The listing builds one solid part. Answer for the finished solid, in the listing's coordinates (mm). Give positions to 0.01 mm unless a question says otherwise; leave off trailing zeros. Write each loop counter-clockwise with the first axis right and the second up, starting at its lowest first coordinate (ties: lowest second). Pieces come first, ordered by that corner, then holes. Notation, with made-up numbers: (46, 44.5) - (103, 44.5) arc R28 cw to (103, 77.5) - close; hole circle Ø10 at (47, 89). An arc over 180 degrees is marked (long way). Answer as CSV lines item,"result". Start each with the question number.
(1) Each of these flat-tipped pins is pushed along its axis until it touches: pin 1 Ø0.7 at (x, z) = (15.5, 2) entering from -Y; pin 2 Ø0.7 at (x, z) = (16, 2) entering from +Y; pin 3 Ø1.5 at (y, z) = (-2.5, 1.5) entering from +X; pin 4 Ø1 at (y, z) = (5.5, 1) entering from -X. Where does it stop, or does it pass through?
(2) Find section B-B (y = -4.75). Write down the section's boundary in (x, z), then the cut area to 3 significant figures.
(3) Straight lines are drawn through the part: probe 1 along X at (y, z) = (1, 1.95); probe 2 along X at (y, z) = (-1, 0.65); probe 3 along Z at (x, y) = (56, -5.5). For each, find the intervals that lie inside material, in ascending order.
(4) Find section A-A (x = 30.5). Write down the section's boundary in (y, z), then the cut area to 3 significant figures.
(5) Find section C-C (x = 48). Write down the section's boundary in (y, z), then the cut area to 3 significant figures.
from build123d import *

# Parameters (mm, degrees)
SKETCH_1_W                      = 90
SKETCH_1_H                      = 15
EXTRUDE_1_DEPTH                 = 2
SKETCH_2_W                      = 3
SKETCH_2_H                      = 3
EXTRUDE_2_DEPTH                 = 1
EXTRUDE_3_DEPTH                 = 2
CUT_EXTRUDE_1_REACH             = 84.878
CUT_EXTRUDE_1_DIRECTION_2_REACH = 84.878
FILLET_1_R                      = 0.1
FILLET_1_OF_MIRROR_1_R          = 0.1
FILLET_1_OF_MIRROR_3_R          = 0.1
FILLET_2_R                      = 0.2


# Read off the part's stored shape, not the designer's step: the mirror step
with BuildPart() as part:
    # Sketch 1 → Extrude 1 (new body)
    with BuildSketch(Plane.XY):
        with Locations((37.5, 0)):
            Rectangle(SKETCH_1_W, SKETCH_1_H)
    extrude(amount=-EXTRUDE_1_DEPTH)

    # Sketch 2 → Extrude 2 (add)
    with BuildSketch(Plane.XY):
        Rectangle(SKETCH_2_W, SKETCH_2_H)
    extrude_2 = extrude(amount=EXTRUDE_2_DEPTH)

    # Sketch 3 → Extrude 3 (add, symmetric)
    with BuildSketch(Plane(origin=(0, 0, 0), x_dir=(1, 0, 0), z_dir=(0, 1, 0))):
        with BuildLine():
            Line((-1.95, -2.5), (1.95, -2.5))
            Line((1.95, -2.5), (1.95, -1.555590279))
            ThreePointArc((1.95, -1.555590279), (1.780042303, -1.088161527), (1.5, -0.677124344))
            Line((1.5, -0.677124344), (-1.5, -0.677124344))
            ThreePointArc((-1.5, -0.677124344), (-1.780042303, -1.088161527), (-1.95, -1.555590279))
            Line((-1.95, -1.555590279), (-1.95, -2.5))
        make_face()
    extrude_3 = extrude(amount=EXTRUDE_3_DEPTH, both=True)

    # Sketch 4 → Cut-Extrude 1 (cut, up to next)
    with BuildSketch(Plane(origin=(0, 0, 0), x_dir=(0, 0, -1), z_dir=(1, 0, 0)), mode=Mode.PRIVATE) as cut_extrude_1_sk1:
        with BuildLine():
            Line((-2.5, 1.95), (-1.555590279, 1.95))
            ThreePointArc((-1.555590279, 1.95), (-1.088161527, 1.780042303), (-0.677124344, 1.5))
            Line((-0.677124344, 1.5), (-0.677124344, 2))
            Line((-0.677124344, 2), (-2.5, 2))
            Line((-2.5, 2), (-2.5, 1.95))
        make_face()
    cut_extrude_1_tool1 = extrude(cut_extrude_1_sk1.sketch, amount=-CUT_EXTRUDE_1_REACH, mode=Mode.PRIVATE) & part.part
    # Sketch 4 → Cut-Extrude 1 (cut, up to next)
    with BuildSketch(Plane(origin=(0, 0, 0), x_dir=(0, 0, -1), z_dir=(1, 0, 0)), mode=Mode.PRIVATE) as cut_extrude_1_sk2:
        with BuildLine():
            Line((-2.5, -2), (-0.677124344, -2))
            Line((-0.677124344, -2), (-0.677124344, -1.5))
            ThreePointArc((-0.677124344, -1.5), (-1.088161527, -1.780042303), (-1.555590279, -1.95))
            Line((-1.555590279, -1.95), (-2.5, -1.95))
            Line((-2.5, -1.95), (-2.5, -2))
        make_face()
    cut_extrude_1_tool2 = extrude(cut_extrude_1_sk2.sketch, amount=-CUT_EXTRUDE_1_REACH, mode=Mode.PRIVATE) & part.part
    cut_extrude_1_1 = cut_extrude_1_tool1.solids().sort_by_distance((0, 1.873038, 1.175075))[0]
    add(cut_extrude_1_1, mode=Mode.SUBTRACT)
    cut_extrude_1_2 = cut_extrude_1_tool2.solids().sort_by_distance((0, -1.873038, 1.175075))[0]
    add(cut_extrude_1_2, mode=Mode.SUBTRACT)
    cut_extrude_1 = cut_extrude_1_1 + cut_extrude_1_2  # Cut-Extrude 1 as one shape, for the pattern or mirror that repeats it

    # Sketch 4 → Cut-Extrude 1 direction 2 (cut, up to next)
    with BuildSketch(Plane(origin=(0, 0, 0), x_dir=(0, 0, -1), z_dir=(1, 0, 0)), mode=Mode.PRIVATE) as cut_extrude_1_direction_2_sk1:
        with BuildLine():
            Line((-2.5, 1.95), (-1.555590279, 1.95))
            ThreePointArc((-1.555590279, 1.95), (-1.088161527, 1.780042303), (-0.677124344, 1.5))
            Line((-0.677124344, 1.5), (-0.677124344, 2))
            Line((-0.677124344, 2), (-2.5, 2))
            Line((-2.5, 2), (-2.5, 1.95))
        make_face()
    cut_extrude_1_direction_2_tool1 = extrude(cut_extrude_1_direction_2_sk1.sketch, amount=CUT_EXTRUDE_1_DIRECTION_2_REACH, mode=Mode.PRIVATE) & part.part
    # Sketch 4 → Cut-Extrude 1 direction 2 (cut, up to next)
    with BuildSketch(Plane(origin=(0, 0, 0), x_dir=(0, 0, -1), z_dir=(1, 0, 0)), mode=Mode.PRIVATE) as cut_extrude_1_direction_2_sk2:
        with BuildLine():
            Line((-2.5, -2), (-0.677124344, -2))
            Line((-0.677124344, -2), (-0.677124344, -1.5))
            ThreePointArc((-0.677124344, -1.5), (-1.088161527, -1.780042303), (-1.555590279, -1.95))
            Line((-1.555590279, -1.95), (-2.5, -1.95))
            Line((-2.5, -1.95), (-2.5, -2))
        make_face()
    cut_extrude_1_direction_2_tool2 = extrude(cut_extrude_1_direction_2_sk2.sketch, amount=CUT_EXTRUDE_1_DIRECTION_2_REACH, mode=Mode.PRIVATE) & part.part
    cut_extrude_1_direction_2_1 = cut_extrude_1_direction_2_tool1.solids().sort_by_distance((0, 1.873038, 1.175075))[0]
    add(cut_extrude_1_direction_2_1, mode=Mode.SUBTRACT)
    cut_extrude_1_direction_2_2 = cut_extrude_1_direction_2_tool2.solids().sort_by_distance((0, -1.873038, 1.175075))[0]
    add(cut_extrude_1_direction_2_2, mode=Mode.SUBTRACT)
    cut_extrude_1_direction_2 = cut_extrude_1_direction_2_1 + cut_extrude_1_direction_2_2  # Cut-Extrude 1 direction 2 as one shape, for the pattern or mirror that repeats it

    # Fillet 1
    fillet_1_edges = [part.edges().sort_by_distance(p)[0] for p in [
        (-1.95, 0, 2.5),
        (1.95, 0, 2.5),
        (0, -1.95, 2.5),
        (0, 1.95, 2.5),
    ]]
    fillet(fillet_1_edges, radius=FILLET_1_R)

    # Mirror 1: Extrude 2, Extrude 3, Cut-Extrude 1, Cut-Extrude 1 direction 2 across plane
    add(extrude_2.mirror(Plane(origin=(7.5, 0, 0), x_dir=(0, 0, 1), z_dir=(1, 0, 0))))
    add(extrude_3.mirror(Plane(origin=(7.5, 0, 0), x_dir=(0, 0, 1), z_dir=(1, 0, 0))))
    add(cut_extrude_1.mirror(Plane(origin=(7.5, 0, 0), x_dir=(0, 0, 1), z_dir=(1, 0, 0))), mode=Mode.SUBTRACT)
    add(cut_extrude_1_direction_2.mirror(Plane(origin=(7.5, 0, 0), x_dir=(0, 0, 1), z_dir=(1, 0, 0))), mode=Mode.SUBTRACT)

    # Fillet 1 of Mirror 1
    fillet_1_of_mirror_1_edges = [part.edges().sort_by_distance(p)[0] for p in [
        (16.95, 0, 2.5),
        (13.05, 0, 2.5),
        (15, -1.95, 2.5),
        (15, 1.95, 2.5),
    ]]
    fillet(fillet_1_of_mirror_1_edges, radius=FILLET_1_OF_MIRROR_1_R)

    # Mirror 3: Extrude 2, Extrude 3, Cut-Extrude 1, Cut-Extrude 1 direction 2 across plane
    add(extrude_2.mirror(Plane(origin=(15, 0, 0), x_dir=(0, 0, 1), z_dir=(1, 0, 0))))
    add(extrude_3.mirror(Plane(origin=(15, 0, 0), x_dir=(0, 0, 1), z_dir=(1, 0, 0))))
    add(cut_extrude_1.mirror(Plane(origin=(15, 0, 0), x_dir=(0, 0, 1), z_dir=(1, 0, 0))), mode=Mode.SUBTRACT)
    add(cut_extrude_1_direction_2.mirror(Plane(origin=(15, 0, 0), x_dir=(0, 0, 1), z_dir=(1, 0, 0))), mode=Mode.SUBTRACT)

    # Fillet 1 of Mirror 3
    fillet_1_of_mirror_3_edges = [part.edges().sort_by_distance(p)[0] for p in [
        (31.95, 0, 2.5),
        (28.05, 0, 2.5),
        (30, -1.95, 2.5),
        (30, 1.95, 2.5),
    ]]
    fillet(fillet_1_of_mirror_3_edges, radius=FILLET_1_OF_MIRROR_3_R)

    # Mirror 4: part across plane


with BuildPart() as part_1:
    add(part.part)
    add(part.part.mirror(Plane(origin=(37.5, 0, 0), x_dir=(0, 0, 1), z_dir=(1, 0, 0))))

    # Fillet 2
    fillet_2_edges = [part_1.edges().sort_by_distance(p)[0] for p in [
        (82.5, 0, -2),
        (37.5, 7.5, -2),
        (-7.5, 0, -2),
        (37.5, 7.5, 0),
        (82.5, 0, 0),
        (37.5, -7.5, 0),
        (-7.5, 0, 0),
        (37.5, -7.5, -2),
        (-7.5, 7.5, -1),
        (82.5, 7.5, -1),
        (82.5, -7.5, -1),
        (-7.5, -7.5, -1),
    ]]
    fillet(fillet_2_edges, radius=FILLET_2_R)


solid = part_1.part
Result set:
1,pin 1,"y = -1.95"
1,pin 2,"y = 1.95"
1,pin 3,"x = 76.95"
1,pin 4,"through"
2,outline,"(-7.5, -1.8) arc R0.2 ccw to (-7.3, -2) - (82.3, -2) arc R0.2 ccw to (82.5, -1.8) - (82.5, -0.2) arc R0.2 ccw to (82.3, 0) - (-7.3, 0) arc R0.2 ccw to (-7.5, -0.2) - close"
2,area,"180 mm^2"
3,probe 1,"-1.95 to 1.95, 13.05 to 16.95, 28.05 to 31.95, 43.05 to 46.95, 58.05 to 61.95, 73.05 to 76.95"
3,probe 2,"-1.5 to 1.5, 13.5 to 16.5, 28.5 to 31.5, 43.5 to 46.5, 58.5 to 61.5, 73.5 to 76.5"
3,probe 3,"-2 to 0"
4,outline,"(-7.5, -1.8) arc R0.2 ccw to (-7.3, -2) - (7.3, -2) arc R0.2 ccw to (7.5, -1.8) - (7.5, -0.2) arc R0.2 ccw to (7.3, 0) - (1.5, 0) - (1.5, 0.68) arc R2 ccw to (1.95, 1.56) - (1.95, 2.4) arc R0.1 ccw to (1.85, 2.5) - (-1.85, 2.5) arc R0.1 ccw to (-1.95, 2.4) - (-1.95, 1.56) arc R2 ccw to (-1.5, 0.68) - (-1.5, 0) - (-7.3, 0) arc R0.2 ccw to (-7.5, -0.2) - close"
4,area,"38.8 mm^2"
5,outline,"(-7.5, -1.8) arc R0.2 ccw to (-7.3, -2) - (7.3, -2) arc R0.2 ccw to (7.5, -1.8) - (7.5, -0.2) arc R0.2 ccw to (7.3, 0) - (-7.3, 0) arc R0.2 ccw to (-7.5, -0.2) - close"
5,area,"30.0 mm^2"
